```python
from build123d import *

# Parameters (mm, degrees)
CROQUIS1_R              = 63
CROQUIS1_R_2            = 60
SALIENTE_EXTRUIR1_DEPTH = 2000
CROQUIS3_W              = 162
CROQUIS3_H              = 220
SALIENTE_EXTRUIR2_DEPTH = 82.5
CROQUIS5_W              = 156
CROQUIS5_H              = 214
CORTAR_EXTRUIR1_DEPTH   = 165


with BuildPart() as part:
    # Croquis1 → Saliente-Extruir1 (new body)
    with BuildSketch(Plane(origin=(44.333451415, -44.333451415, 0), x_dir=(0, 0, -1), z_dir=(0.7071067811865438, -0.7071067811865512, 0))):
        with Locations(Location((27.566313026, 62.696968258, 0), (0, 0, 90))):
            Circle(CROQUIS1_R)
        with Locations(Location((27.566313026, 62.696968258, 0), (0, 0, 90))):
            Circle(CROQUIS1_R_2, mode=Mode.SUBTRACT)
    extrude(amount=-SALIENTE_EXTRUIR1_DEPTH)

    # Croquis3 → Saliente-Extruir2 (add, symmetric)
    with BuildSketch(Plane(origin=(44.333451415, 44.333451415, 0), x_dir=(0, 0, -1), z_dir=(0.7071067811865488, 0.7071067811865464, 0))):
        with Locations((27.566313026, 1707.303031742)):
            Rectangle(CROQUIS3_W, CROQUIS3_H)
    extrude(amount=SALIENTE_EXTRUIR2_DEPTH, both=True)

    # Croquis5 → Cortar-Extruir1 (cut)
    with BuildSketch(Plane(origin=(102.669760863, 102.669760863, 0), x_dir=(0, 0, -1), z_dir=(0.7071067811865485, 0.7071067811865467, 0))):
        with Locations((27.566313026, 1707.303031742)):
            Rectangle(CROQUIS5_W, CROQUIS5_H)
    extrude(amount=-CORTAR_EXTRUIR1_DEPTH, mode=Mode.SUBTRACT)


solid = part.part
```
Geometry check sheet. Reference: the model listing, model coordinates, mm. A direction names the side the tool comes from. Coordinates: 2 decimals unless noted, no trailing zeros. Order: outer loops, then holes, each group sorted by start corner. A loop starts at its lowest first (then second) coordinate and runs counter-clockwise, first axis right, second up. Notation, with made-up numbers: (-23.75, -15) - (-16.75, -15) arc R33 ccw to (-16.75, 24) - close; hole circle Ø9 at (50.25, 32). An arc over 180 degrees is marked (long way). Use one line per item in the form item = value.
1. Gauge pin test, flat ends, axial feed: pin 1 (8 mm diameter, centred on y = 414, z = 18, fed in from -X); pin 2 (5 mm diameter, centred on x = -611.5, z = -75.5, fed in from -Y); pin 3 (1 mm diameter, centred on x = -157, z = -3, fed in from -Y). Record the tip position at first contact, or that the pin passes through.
Here are the results:
pin_1 = -393.67
pin_2 = 637.68
pin_3 = 163.04
2. Access from +Z, -Z, +X, -X, +Y, -Y to the whole of each face (thin tool, end or side, straight path). Record for faces 1 (the face through (-1086.43, 1176.74, -26.47)), 2 (the face through (-1104.94, 1310.28, 50.81)), 3 (the face through (-1161, 1251, 50.434)).
Here are the results:
face_1 = -X, +Y
face_2 = +Z, -Z, +X, +Y
face_3 = none
3. Scan lines: line 1 (Z direction, x = -1136.5, y = 1234); line 2 (X direction, y = 986, z = 22); line 3 (X direction, y = 1384.5, z = 0). Record each from-to range of solid material in increasing order.
Here are the results:
line_1 = -108.57 to -105.57, 50.43 to 53.43
line_2 = -952.33 to -945.15, -849.52 to -842.34
line_3 = -1220.47 to -1215.72, -1185.55 to -1181.31
4. Section check A-A (z = 11). Record the boundary of the cut face in (x, y).
Here are the results:
outline = (-1360.77, 1378.99) - (-1275.92, 1294.14) - (-1299.03, 1271.02) - (-1296.91, 1268.9) - (-1180.24, 1385.58) - (-1182.36, 1387.7) - (-1205.47, 1364.59) - (-1290.32, 1449.44) - (-1293.05, 1446.71) - (-1208.19, 1361.86) - (-1273.19, 1296.86) - (-1358.05, 1381.71) - close; (-1145.59, 1117.58) - (-1143.47, 1115.46) - (-1120.36, 1138.57) - (53.44, -35.23) - (56.17, -32.5) - (-1117.63, 1141.3) - (-1052.63, 1206.3) - (121.17, 32.5) - (123.89, 35.23) - (-1049.91, 1209.02) - (-1026.79, 1232.13) - (-1028.92, 1234.25) - close
5. Draft check along X on faces 4 (the face through (-1286.16, 1453.6, -50.61)), 5 (the face through (-1213.95, 1356.105, 27.568)), 6 (the face through (-1237.756, 1328.056, -26.474)), 7 (the face through (-1084.54, 1174.39, -26.73)). Enter one of: pulls with the +X half, pulls with the -X half, needs draft (parallel to the pull), parting line crosses it, or undercut.
Here are the results:
face_4 = pulls with the -X half
face_5 = undercut
face_6 = pulls with the +X half
face_7 = undercut
